```python
from build123d import *

# Parameters (mm, degrees)
SKETCH1_W           = 60
SKETCH1_H           = 43
BOSS_EXTRUDE1_DEPTH = 5
SKETCH2_W           = 60
SKETCH2_H           = 5
BOSS_EXTRUDE2_DEPTH = 4.4
SKETCH3_W           = 3
SKETCH3_H           = 43
BOSS_EXTRUDE3_DEPTH = 6.4
SKETCH4_W           = 43
SKETCH4_H           = 3
BOSS_EXTRUDE4_DEPTH = 2.3
SKETCH5_W           = 30
SKETCH5_H           = 56
BOSS_EXTRUDE5_DEPTH = 28.5
SKETCH6_W           = 40.4
SKETCH6_H           = 20.4
CUT_EXTRUDE1_DEPTH  = 28
SKETCH7_R           = 1.05
CUT_EXTRUDE2_DEPTH  = 25
CUT_EXTRUDE3_REACH  = 94.427
SKETCH8_W           = 5.4
SKETCH8_H           = 3
CUT_EXTRUDE4_REACH  = 92.735
SKETCH9_R           = 1.7
SKETCH10_R          = 3
CUT_EXTRUDE5_DEPTH  = 3


with BuildPart() as part:
    # Sketch1 → Boss-Extrude1 (new body)
    with BuildSketch(Plane(origin=(0, 0, 0), x_dir=(1, 0, 0), z_dir=(0, 1, 0))):
        with Locations((30, 21.5)):
            Rectangle(SKETCH1_W, SKETCH1_H)
    extrude(amount=BOSS_EXTRUDE1_DEPTH)

    # Sketch2 → Boss-Extrude2 (add)
    with BuildSketch(Plane(origin=(0, 0, 0), x_dir=(-1, 0, 0), z_dir=(0, -1, 0))):
        with Locations((-30, 2.5)):
            Rectangle(SKETCH2_W, SKETCH2_H)
        with Locations((-30, 40.5)):
            Rectangle(SKETCH2_W, SKETCH2_H)
    extrude(amount=BOSS_EXTRUDE2_DEPTH)

    # Sketch3 → Boss-Extrude3 (add)
    with BuildSketch(Plane(origin=(0, 5, 0), x_dir=(1, 0, 0), z_dir=(0, 1, 0))):
        with Locations((6.5, 21.5)):
            Rectangle(SKETCH3_W, SKETCH3_H)
        with Locations((19.5, 21.5)):
            Rectangle(SKETCH3_W, SKETCH3_H)
    extrude(amount=BOSS_EXTRUDE3_DEPTH)

    # Sketch4 → Boss-Extrude4 (add)
    with BuildSketch(Plane(origin=(8, 0, 0), x_dir=(0, 0, -1), z_dir=(1, 0, 0))):
        with Locations((21.5, 9.9)):
            Rectangle(SKETCH4_W, SKETCH4_H)
    boss_extrude4 = extrude(amount=BOSS_EXTRUDE4_DEPTH)

    # Mirror1: Boss-Extrude4 across plane
    add(boss_extrude4.mirror(Plane(origin=(13, 0, 0), x_dir=(0, 0, 1), z_dir=(1, 0, 0))))

    # Sketch5 → Boss-Extrude5 (add)
    with BuildSketch(Plane(origin=(0, 5, 0), x_dir=(1, 0, 0), z_dir=(0, 1, 0))):
        with Locations((55.5, 21.5)):
            Rectangle(SKETCH5_W, SKETCH5_H)
    extrude(amount=BOSS_EXTRUDE5_DEPTH)

    # Sketch6 → Cut-Extrude1 (cut)
    with BuildSketch(Plane.ZY.offset(-40.5)):
        with Locations((-21.5, 20.5)):
            Rectangle(SKETCH6_W, SKETCH6_H)
    extrude(amount=-CUT_EXTRUDE1_DEPTH, mode=Mode.SUBTRACT)

    # Sketch7 → Cut-Extrude2 (cut)
    with BuildSketch(Plane.ZY.offset(-40.5)):
        with Locations((-46, 25.5)):
            Circle(SKETCH7_R)
        with Locations((-46, 15.5)):
            Circle(SKETCH7_R)
        with Locations((3, 25.5)):
            Circle(SKETCH7_R)
        with Locations((3, 15.5)):
            Circle(SKETCH7_R)
    extrude(amount=-CUT_EXTRUDE2_DEPTH, mode=Mode.SUBTRACT)

    # Sketch8 → Cut-Extrude3 (cut, up to next)
    with BuildSketch(Plane.XY, mode=Mode.PRIVATE) as cut_extrude3_sk1:
        with Locations((13, 3.5)):
            Rectangle(SKETCH8_W, SKETCH8_H)
    cut_extrude3_tool1 = extrude(cut_extrude3_sk1.sketch, amount=-CUT_EXTRUDE3_REACH, mode=Mode.PRIVATE) & part.part
    add(cut_extrude3_tool1.solids().sort_by_distance((13, 3.5, 0))[0], mode=Mode.SUBTRACT)

    # Sketch9 → Cut-Extrude4 (cut, up to next)
    with BuildSketch(Plane(origin=(0, 5, 0), x_dir=(1, 0, 0), z_dir=(0, 1, 0)), mode=Mode.PRIVATE) as cut_extrude4_sk1:
        with Locations(Location((26.5, 40.5, 0), (0, 0, 270))):
            Circle(SKETCH9_R)
    cut_extrude4_tool1 = extrude(cut_extrude4_sk1.sketch, amount=-CUT_EXTRUDE4_REACH, mode=Mode.PRIVATE) & part.part
    # Sketch9 → Cut-Extrude4 (cut, up to next)
    with BuildSketch(Plane(origin=(0, 5, 0), x_dir=(1, 0, 0), z_dir=(0, 1, 0)), mode=Mode.PRIVATE) as cut_extrude4_sk2:
        with Locations(Location((36.5, 40.5, 0), (0, 0, 270))):
            Circle(SKETCH9_R)
    cut_extrude4_tool2 = extrude(cut_extrude4_sk2.sketch, amount=-CUT_EXTRUDE4_REACH, mode=Mode.PRIVATE) & part.part
    # Sketch9 → Cut-Extrude4 (cut, up to next)
    with BuildSketch(Plane(origin=(0, 5, 0), x_dir=(1, 0, 0), z_dir=(0, 1, 0)), mode=Mode.PRIVATE) as cut_extrude4_sk3:
        with Locations(Location((36.5, 2.5, 0), (0, 0, 90))):
            Circle(SKETCH9_R)
    cut_extrude4_tool3 = extrude(cut_extrude4_sk3.sketch, amount=-CUT_EXTRUDE4_REACH, mode=Mode.PRIVATE) & part.part
    # Sketch9 → Cut-Extrude4 (cut, up to next)
    with BuildSketch(Plane(origin=(0, 5, 0), x_dir=(1, 0, 0), z_dir=(0, 1, 0)), mode=Mode.PRIVATE) as cut_extrude4_sk4:
        with Locations(Location((26.5, 2.5, 0), (0, 0, 90))):
            Circle(SKETCH9_R)
    cut_extrude4_tool4 = extrude(cut_extrude4_sk4.sketch, amount=-CUT_EXTRUDE4_REACH, mode=Mode.PRIVATE) & part.part
    add(cut_extrude4_tool1.solids().sort_by_distance((26.5, 5, -40.5))[0], mode=Mode.SUBTRACT)
    add(cut_extrude4_tool2.solids().sort_by_distance((36.5, 5, -40.5))[0], mode=Mode.SUBTRACT)
    add(cut_extrude4_tool3.solids().sort_by_distance((36.5, 5, -2.5))[0], mode=Mode.SUBTRACT)
    add(cut_extrude4_tool4.solids().sort_by_distance((26.5, 5, -2.5))[0], mode=Mode.SUBTRACT)

    # Sketch10 → Cut-Extrude5 (cut)
    with BuildSketch(Plane(origin=(0, 5, 0), x_dir=(1, 0, 0), z_dir=(0, 1, 0))):
        with Locations((26.5, 40.5)):
            Circle(SKETCH10_R)
        with Locations((36.5, 40.5)):
            Circle(SKETCH10_R)
        with Locations((26.5, 2.5)):
            Circle(SKETCH10_R)
        with Locations((36.5, 2.5)):
            Circle(SKETCH10_R)
    extrude(amount=-CUT_EXTRUDE5_DEPTH, mode=Mode.SUBTRACT)


solid = part.part
```
Geometry check sheet. Reference: the model listing, model coordinates, mm. A direction names the side the tool comes from. Round coordinates to 2 decimals unless told otherwise and drop trailing zeros. Loops run counter-clockwise (first coordinate to the right, second up) from the corner with the lowest first, then second, coordinate; pieces in that order, holes last. Notation, with made-up numbers: (-19.75, 64.5) - (-10.75, 64.5) arc R35 cw to (-10.75, 100.5) - close; hole circle Ø7 at (47, 54.5). An arc over 180 degrees is marked (long way). Use a Markdown table: item, result.
Q1. Draft check along Y on faces 4 (the flat face through (30, 0, -22)), 5 (the cylindrical face through (36.6, 3.5, -5.5)), 6 (the cylindrical face through (52.825, 24.475, 2.772)), 7 (the flat face through (38, 2, -4)). Enter one of: released by +Y, released by -Y, zero draft, split by the parting line, or undercut.
Solutions:
| item | result |
|---|---|
| face 4 | released by -Y |
| face 5 | zero draft |
| face 6 | undercut |
| face 7 | released by +Y |
Q2. Cross-section at D-D on x = 26.5. Record the cut outline in (y, z).
Solutions:
| item | result |
|---|---|
| outline | (-4.4, -43) - (2, -43) - (2, -42.2) - (-4.4, -42.2) - close; (-4.4, -38.8) - (2, -38.8) - (2, -37.5) - (5, -37.5) - (5, -5.5) - (2, -5.5) - (2, -4.2) - (-4.4, -4.2) - (-4.4, -5) - (0, -5) - (0, -38) - (-4.4, -38) - close; (-4.4, -0.8) - (2, -0.8) - (2, 0) - (-4.4, 0) - close |
Q3. Go/stop test with flat-tipped pins: P1, Ø10, axis at x = 29, z = -28.5, coming from the +Y side; P2, Ø2.5, axis at x = 8.5, z = -29, coming from the +Y side; P3, Ø2, axis at y = 11.5, z = -20.5, coming from the -X side. Record where each tip stops, or that it passes through.
Solutions:
| item | result |
|---|---|
| P1 | stops at y = 5 |
| P2 | stops at y = 11.4 |
| P3 | stops at x = 5 |
Q4. Material ranges on line 1 (Y direction, x = 57, z = 3); line 2 (X direction, y = -0.5, z = -40.5); line 3 (X direction, y = 10.5, z = -39), recorded low to high.
Solutions:
| item | result |
|---|---|
| line 1 | y = 5 to 14.45, 16.55 to 24.45, 26.55 to 33.5 |
| line 2 | x = 0 to 24.8, 28.2 to 34.8, 38.2 to 60 |
| line 3 | x = 5 to 10.3, 15.7 to 21, 68.5 to 70.5 |
Q5. Cross-section at B-B on x = 16.5. Record the cut outline in (y, z), plus the area to 3 significant figures.
Solutions:
| item | result |
|---|---|
| outline | (-4.4, -43) - (5, -43) - (5, 0) - (-4.4, 0) - (-4.4, -5) - (0, -5) - (0, -38) - (-4.4, -38) - close; (8.4, -43) - (11.4, -43) - (11.4, 0) - (8.4, 0) - close |
| area | 388 mm2 |
Q6. Cross-section at A-A on y = -2. Record the cut outline in (x, z), plus the area to 3 significant figures.
Solutions:
| item | result |
|---|---|
| outline | (0, -43) - (60, -43) - (60, -38) - (0, -38) - close; (0, -5) - (60, -5) - (60, 0) - (0, 0) - close; hole circle Ø3.4 at (26.5, -40.5); hole circle Ø3.4 at (26.5, -2.5); hole circle Ø3.4 at (36.5, -40.5); hole circle Ø3.4 at (36.5, -2.5) |
| area | 564 mm2 |
Q7. Cross-section at C-C on z = -10. Record the cut outline in (x, y), plus the area to 3 significant figures.
Solutions:
| item | result |
|---|---|
| outline | (0, 0) - (60, 0) - (60, 5) - (70.5, 5) - (70.5, 33.5) - (40.5, 33.5) - (40.5, 30.7) - (68.5, 30.7) - (68.5, 10.3) - (40.5, 10.3) - (40.5, 5) - (21, 5) - (21, 11.4) - (15.7, 11.4) - (15.7, 8.4) - (18, 8.4) - (18, 5) - (15.7, 5) - (15.7, 2) - (10.3, 2) - (10.3, 5) - (8, 5) - (8, 8.4) - (10.3, 8.4) - (10.3, 11.4) - (5, 11.4) - (5, 5) - (0, 5) - close |
| area | 620 mm2 |
Q8. Access from +Z, -Z, +X, -X, +Y, -Y to the whole of each face (thin tool, end or side, straight path). Record for faces 1 (the flat face through (17, 5, -22)), 2 (the flat face through (2, 5, -22)), 3 (the flat face through (21, 8, -21)).
Solutions:
| item | result |
|---|---|
| face 1 | +Z, -Z |
| face 2 | +Z, -Z, -X, +Y |
| face 3 | +Z, -Z, +Y |
